Study the drawing (mm; zero at the part's minimum x, y, z) and answer. Coordinates: 2 decimals unless noted, no trailing zeros. Write each loop counter-clockwise with the first axis right and the second up, starting at its lowest first coordinate (ties: lowest second). Pieces come first, ordered by that corner, then holes. Notation, with made-up numbers: M -23.5,17.5 L 14.5,17.5 A29 ccw 14.5,43.5 Z; hole C 9,72.25 d9. An arc over 180 degrees is marked long. Answer as a JSON object with one key per item and string values. Group by question number.
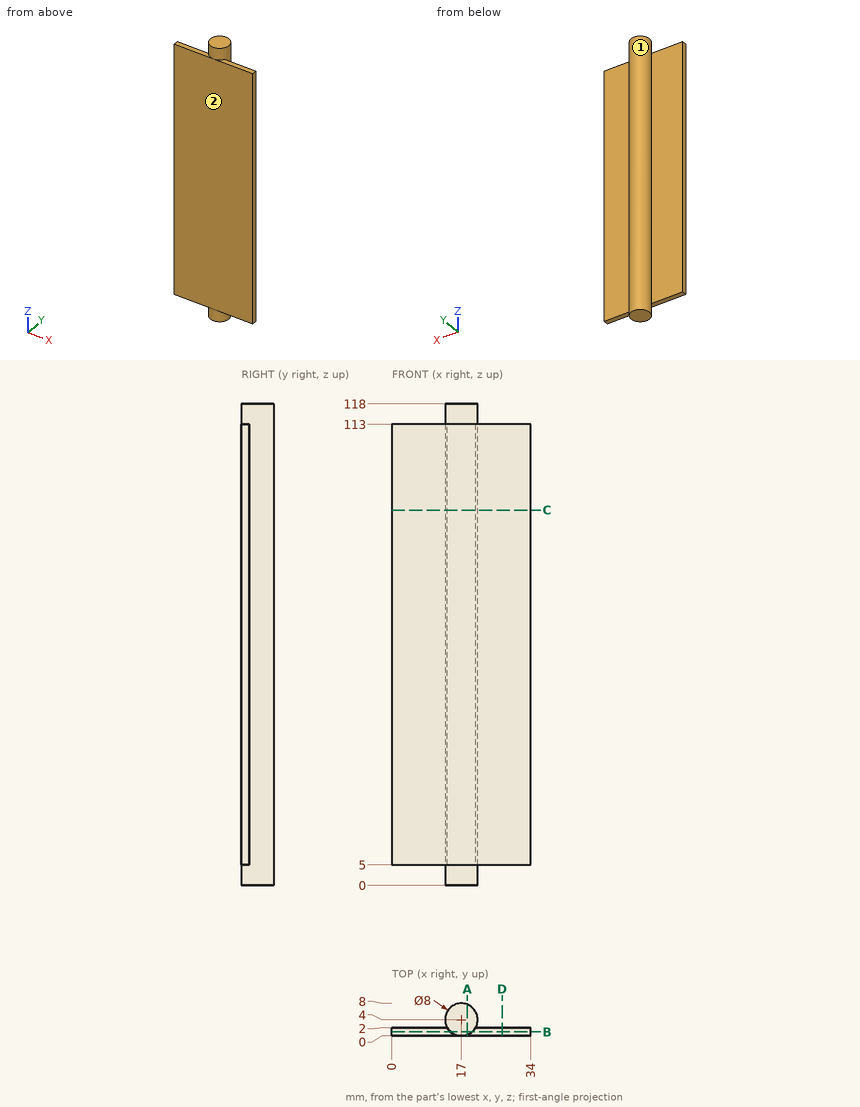
Item 1: A cutting plane is placed at A-A, the plane x = 18.5. Write down the section's boundary in (y, z).
Item 2: Consider L1, parallel to Y at x = 33.5, z = 57.5; L2, parallel to Z at x = 21.5, y = 0.5; L3, parallel to X at y = 4.25, z = 26. Determine where each line is inside the solid, lowest interval first. Write a range as from..to.
Item 3: For a pull along Y with two mould halves and no side action, classify the marked faces 1 and 2 as +Y half, -Y half, draft (parallel to the pull), parting line (faces both ways), or undercut.
Item 4: A cutting plane is placed at C-C, the plane z = 92. Write down the section's boundary in (x, y).
Item 5: Flat-ended cylindrical pins translate along their axes: pin 1 Ø1 at (x, y) = (25.5, 1) entering from +Z; pin 2 Ø1.5 at (y, z) = (4, 32) entering from +X; pin 3 Ø4 at (x, y) = (26, 1) entering from -Z. Find the tip coordinate at first contact, or state that the pin passes through.
Item 6: A cutting plane is placed at B-B, the plane y = 1. Write down the section's boundary in (x, z), and give its area (3 significant figures).
Item 7: A cutting plane is placed at D-D, the plane x = 27. Write down the section's boundary in (y, z), and give its area (3 significant figures).
Answer:
{
 "1": {"outline": "M 0,5 L 0.29,5 L 0.29,0 L 7.71,0 L 7.71,118 L 0.29,118 L 0.29,113 L 0,113 Z"},
 "2": {"L1": "0..2", "L2": "5..113", "L3": "13.01..20.99"},
 "3": {"face 1": "undercut", "face 2": "-Y half"},
 "4": {"outline": "M 0,0 L 34,0 L 34,2 L 20.46,2 A4 ccw long 13.54,2 L 0,2 Z"},
 "5": {"pin 1": "z = 113", "pin 2": "x = 21", "pin 3": "z = 5"},
 "6": {"outline": "M 0,5 L 14.35,5 L 14.35,0 L 19.65,0 L 19.65,5 L 34,5 L 34,113 L 19.65,113 L 19.65,118 L 14.35,118 L 14.35,113 L 0,113 Z", "area": "3,720 mm2"},
 "7": {"outline": "M 0,5 L 2,5 L 2,113 L 0,113 Z", "area": "216 mm2"}
}
